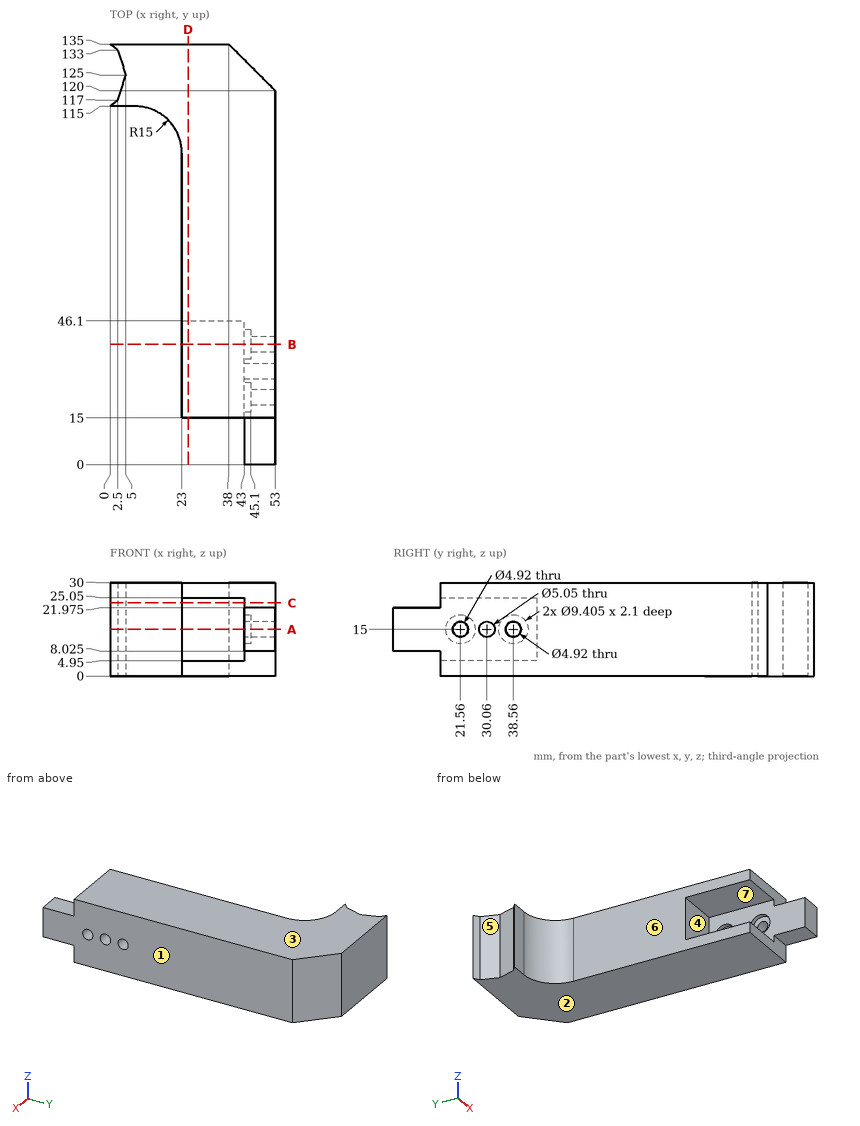
Check sheet for the drawn part. Datum: minimum x, y, z corner. Units: mm. A direction names the side the tool comes from. Round coordinates to 2 decimals unless told otherwise and drop trailing zeros. Write each loop counter-clockwise with the first axis right and the second up, starting at its lowest first coordinate (ties: lowest second). Pieces come first, ordered by that corner, then holes. Notation, with made-up numbers: (-28, -21) - (-8, -21) arc R18 ccw to (-8, 6) - close; hole circle Ø2 at (68, -20.5). An arc over 180 degrees is marked (long way). Return JSON: item names as keys, results as strings.
Q1. Cross-section at A-A (z = 15). Give the number of separate pieces and of enclosed holes in the cut face, then the cut area to 3 significant figures.
Returned:
{"separate pieces": "4", "enclosed holes": "0", "area": "3,290 mm²"}
Q2. Draft check along Z on the marked faces 1, 2, 3 and 4. Enter one of: released by +Z, released by -Z, zero draft, split by the parting line, or undercut.
Returned:
{"face 1": "zero draft", "face 2": "released by -Z", "face 3": "released by +Z", "face 4": "undercut"}
Q3. Cross-section at B-B (y = 38.56). Record the boundary of the cut face in (x, z).
Returned:
{"outline": "(23, 0) - (53, 0) - (53, 12.54) - (45.1, 12.54) - (45.1, 10.3) - (43, 10.3) - (43, 4.95) - (23, 4.95) - close; (23, 25.05) - (43, 25.05) - (43, 19.7) - (45.1, 19.7) - (45.1, 17.46) - (53, 17.46) - (53, 30) - (23, 30) - close"}
Q4. Scan lines: L1, parallel to Y at x = 47.75, z = 15 (3 decimals); L2, parallel to Y at x = 48.5, z = 15 (3 decimals); L3, parallel to X at y = 14, z = 20. Record each from-to range of solid material in increasing order. Write a range as from..to.
Returned:
{"L1": "y = 0..19.1, 24.02..27.535, 32.585..36.1, 41.02..125.25", "L2": "y = 0..19.1, 24.02..27.535, 32.585..36.1, 41.02..124.5", "L3": "x = 43..53"}
Q5. Depth check by flat-ended pin: P1, Ø10.5, axis at y = 20, z = 17, coming from the -X side; P2, Ø4, axis at x = 39, z = 23, coming from the +Y side; P3, Ø4.5, axis at y = 21.56, z = 15, coming from the +X side (3 decimals); P4, Ø2.5, axis at x = 5, z = 16.5, coming from the -Y side. Enter the tip coordinate at first touch or a pass-through.
Returned:
{"P1": "stops at x = 43", "P2": "stops at y = 135", "P3": "passes through", "P4": "stops at y = 115"}
Q6. Cross-section at D-D (x = 25). Record the boundary of the cut face in (y, z).
Returned:
{"outline": "(15, 0) - (135, 0) - (135, 30) - (15, 30) - (15, 25.05) - (46.1, 25.05) - (46.1, 4.95) - (15, 4.95) - close"}
Q7. Access from +Z, -Z, +X, -X, +Y, -Y to the whole of each face (thin tool, end or side, straight path). Record for the marked faces 5, 6 and 7.
Returned:
{"face 5": "+Z, -Z, -X", "face 6": "+Z, -Z, -X, -Y", "face 7": "-X, -Y"}
Q8. Cross-section at C-C (z = 23.5). Record the boundary of the cut face in (x, y), then the cut area to 3 significant figures.
Returned:
{"outline": "(0, 115) - (8, 115) arc R15 cw to (23, 100) - (23, 46.1) - (43, 46.1) - (43, 15) - (53, 15) - (53, 120) - (38, 135) - (0, 135) - (2.5, 133) - (5, 125) - (2.5, 117) - close", "area": "3,310 mm²"}
